Source: three-view drawing plus pictorial views. Frame: mm from the lowest corner of the part. A direction names the side the tool comes from. Round coordinates to 2 decimals unless told otherwise and drop trailing zeros. Loops run counter-clockwise (first coordinate to the right, second up) from the corner with the lowest first, then second, coordinate; pieces in that order, holes last. Notation, with made-up numbers: (-2, 8.25) -> (6, 8.25) arc R29 ccw to (6, 37.25) -> close; hole circle Ø6 at (-4.75, -7). An arc over 180 degrees is marked (long way). Answer in a Markdown table with one row per item. Add a question column.
Q1. Pin query (flat end, axial travel): pin 1 (1.5 mm diameter, centred on y = 11, z = 1.5, fed in from +X); pin 2 (1.5 mm diameter, centred on x = 19.5, y = 11, fed in from +Z); pin 3 (1 mm diameter, centred on y = 6, z = 7, fed in from -X). Return the tip coordinate at first contact, or that it passes through.
Q2. Ray query, L1, parallel to X at y = 5.5, z = 3.25; L2, parallel to X at y = 4.5, z = 0.75; L3, parallel to X at y = 16.25, z = 7. Return the intervals inside material, ascending. Write a range as from..to.
Q3. Section C-C, the plane y = 4.75. Output: boundary loops of the cut face in (x, z).
Q4. Reachability of the marked faces 1, 2, 3, 4 and 5 from +Z, -Z, +X, -X, +Y, -Y: full face, straight path, thin tool, end or side. Return the list, or none.
Q5. Section A-A, the plane y = 12. Output: boundary loops of the cut face in (x, z), and give its area (3 significant figures).
Q6. Mould query, pull axis X, two halves, no side actions, for the marked faces 6, 7 and 8. Classes: pulls with the +X half, pulls with the -X half, needs draft (parallel to the pull), parting line crosses it, or undercut.
Q7. Section D-D, the plane x = 10.5. Output: boundary loops of the cut face in (y, z), and give its area (4 significant figures).
Q8. Section B-B, the plane z = 5.5. Output: boundary loops of the cut face in (x, y).
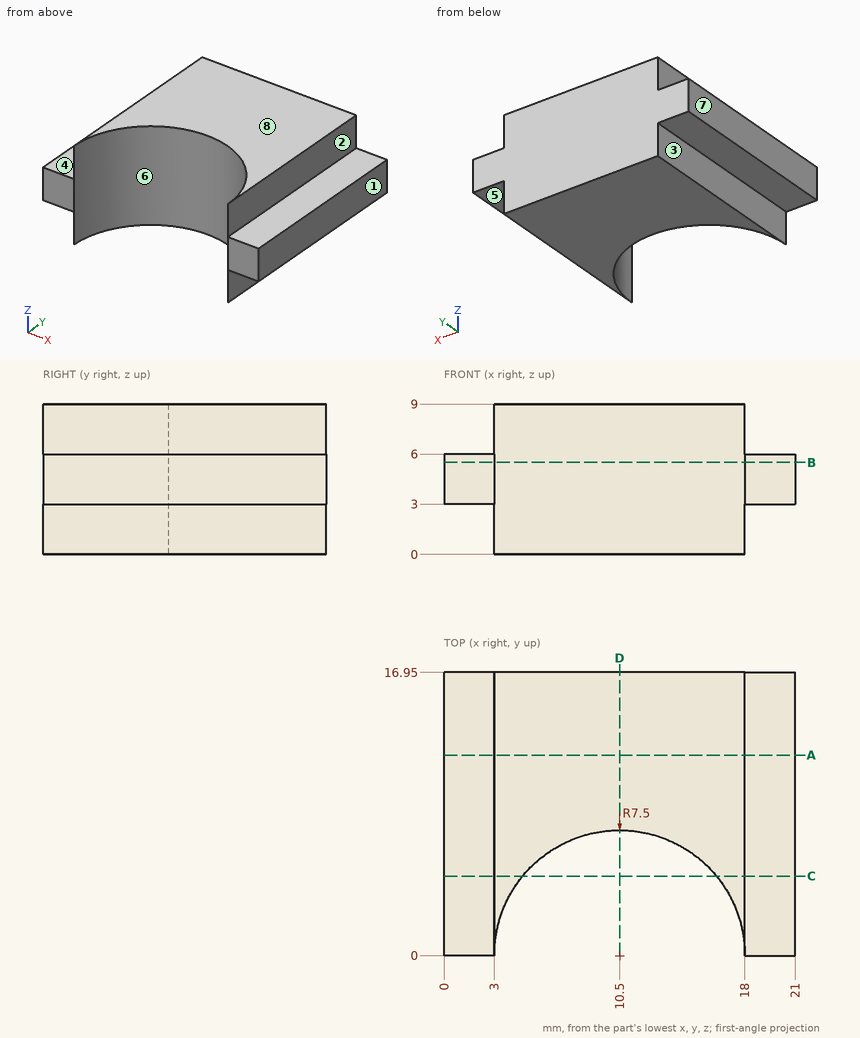
Answer block:
| question | item | result |
|---|---|---|
| 1 | pin 1 | x = 18 |
| 1 | pin 2 | z = 6 |
| 1 | pin 3 | x = 3 |
| 2 | L1 | 0..5.4, 15.6..21 |
| 2 | L2 | 3..4.5, 16.5..18 |
| 2 | L3 | 3..18 |
| 3 | outline | (0, 3) -> (3, 3) -> (3, 0) -> (4.7, 0) -> (4.7, 9) -> (3, 9) -> (3, 6) -> (0, 6) -> close; (16.3, 0) -> (18, 0) -> (18, 3) -> (21, 3) -> (21, 6) -> (18, 6) -> (18, 9) -> (16.3, 9) -> close |
| 4 | face 1 | +Z, -Z, +X, +Y, -Y |
| 4 | face 2 | +Z, +X, +Y, -Y |
| 4 | face 3 | -Z, -X, +Y, -Y |
| 4 | face 4 | +Z, -X, +Y, -Y |
| 4 | face 5 | -Z, +X, +Y, -Y |
| 5 | outline | (0, 3) -> (3, 3) -> (3, 0) -> (18, 0) -> (18, 3) -> (21, 3) -> (21, 6) -> (18, 6) -> (18, 9) -> (3, 9) -> (3, 6) -> (0, 6) -> close |
| 5 | area | 153 mm^2 |
| 6 | face 6 | undercut |
| 6 | face 7 | pulls with the -X half |
| 6 | face 8 | needs draft |
| 7 | outline | (7.5, 0) -> (16.95, 0) -> (16.95, 9) -> (7.5, 9) -> close |
| 7 | area | 85.05 mm^2 |
| 8 | outline | (0, 0) -> (3, 0) arc R7.5 cw to (18, 0) -> (21, 0) -> (21, 16.95) -> (0, 16.95) -> close |
